CAD build for the part. Positions are in the model's coordinates, mm. A direction names the side the tool comes from. Coordinates: 2 decimals unless noted, no trailing zeros. Loops run counter-clockwise (first coordinate to the right, second up) from the corner with the lowest first, then second, coordinate; pieces in that order, holes last. Notation, with made-up numbers: (-8.75, 21.25) -> (19.25, 21.25) arc R32 ccw to (19.25, 50.25) -> close; hole circle Ø6 at (-32.75, 0). An arc over 180 degrees is marked (long way). Write item = value, one per line. Start each with the question number.
(1) Pull direction Z, two halves, no side cores. Call faces 1 (the face through (3, 6, -8.746)), 2 (the face through (4, 6, -12)), 3 (the face through (4, 0, -13.246)): +Z half, -Z half, draft (parallel to the pull), parting line (faces both ways), or undercut.
(2) Drill centre lines: line 1 (X direction, y = -2, z = -0.75); line 2 (X direction, y = -1.5, z = -3.25); line 3 (Z direction, x = 6, y = 5.5). Where is each one in solid material? Low to high. Write a range as from..to.
(3) Band-saw the part on B-B (x = 3). Write the cut outline in (y, z).
(4) Band-saw the part on D-D (y = -2). Write the cut outline in (x, z).
(5) Band-saw the part on A-A (y = 5.75). Write the cut outline in (x, z).
(6) Flat gauge pins, fed straight in: P1, Ø5, axis at y = -4.5, z = -3, coming from the -X side; P2, Ø1, axis at y = -1, z = -8.5, coming from the -X side; P3, Ø4, axis at x = 11.5, y = 0, coming from the -Z side; P4, Ø1, axis at x = 3, z = -9.5, coming from the +Y side. Where does each tip first touch, or does it go through?
(7) Tool access for faces 4 (the face through (17.5, 0, -1)), 5 (the face through (2, 0, -7)), 6 (the face through (6, 0, -11)), 7 (the face through (8, 0, 0)), 8 (the face through (3, -6, -11.246)): list every direction of +Z, -Z, +X, -X, +Y, -Y with a clear straight run to the whole face (end or side of a thin tool).
(8) Band-saw the part on C-C (z = -9.25). Write the cut outline in (x, y) (1 decimal), and give its area (3 significant figures).
```python
from build123d import *

# Parameters (mm, degrees)
BOSS_EXTRUDE1_DEPTH = 7.5
SKETCH2_W           = 2.5
SKETCH2_H           = 3
CUT_EXTRUDE2_DEPTH  = 20
BOSS_EXTRUDE2_REACH = 16


with BuildPart() as part:
    # Sketch1 → Boss-Extrude1 (new body, symmetric)
    with BuildSketch(Plane(origin=(0, 0, 0), x_dir=(1, 0, 0), z_dir=(0, 1, 0))):
        Polygon((2, 13.245621125), (2, 1.5), (0, 1.5), (0, 0), (15.5, 0), (15.5, -0.754378875), (17.5, -0.754378875), (17.5, 1.128157441), (17.5, 2.995621125), (19, 2.995621125), (19, 4.67916542), (4, 8.745621125), (4, 13.245621125), align=None)
    extrude(amount=BOSS_EXTRUDE1_DEPTH, both=True)

    # Sketch2 → Cut-Extrude2 (cut, through all)
    with BuildSketch(Plane(origin=(0, 0, 0), x_dir=(0, 0, -1), z_dir=(1, 0, 0))):
        with Locations((9.995621125, 6)):
            Rectangle(SKETCH2_W, SKETCH2_H)
        with Locations((9.995621125, -6)):
            Rectangle(SKETCH2_W, SKETCH2_H)
    extrude(amount=CUT_EXTRUDE2_DEPTH, mode=Mode.SUBTRACT)

    # Boss-Extrude2: up to this face of the body (flat: up to its plane)
    boss_extrude2_end = Plane(part.part.faces().sort_by_distance((11.5, 0, -6.712393272))[0])
    # Sketch4 → Boss-Extrude2 (add, up to the picked face)
    with BuildSketch(Plane(origin=(0, 0, -13.245621125), x_dir=(-1, 0, 0), z_dir=(0, 0, -1)), mode=Mode.PRIVATE) as boss_extrude2_sk1:
        with BuildLine():
            Line((-4, 4.5), (-4, -4.5))
            ThreePointArc((-4, -4.5), (-6, 0), (-4, 4.5))
        make_face()
    boss_extrude2_tool1 = split(extrude(boss_extrude2_sk1.sketch, amount=-BOSS_EXTRUDE2_REACH, mode=Mode.PRIVATE), bisect_by=boss_extrude2_end, keep=Keep.BOTH, mode=Mode.PRIVATE)
    add(boss_extrude2_tool1.solids().sort_by_distance((4.812513, 0, -13.245621))[0])


solid = part.part
```
Findings below:
q1.face_1 = undercut
q1.face_2 = draft
q1.face_3 = -Z half
q2.line_1 = 0..17.5
q2.line_2 = 2..19
q2.line_3 = -8.2..0
q3.outline = (-7.5, -13.25) -> (7.5, -13.25) -> (7.5, -11.25) -> (4.5, -11.25) -> (4.5, -8.75) -> (7.5, -8.75) -> (7.5, 0) -> (-7.5, 0) -> (-7.5, -8.75) -> (-4.5, -8.75) -> (-4.5, -11.25) -> (-7.5, -11.25) -> close
q4.outline = (0, -1.5) -> (2, -1.5) -> (2, -13.25) -> (5.66, -13.25) -> (5.66, -8.3) -> (19, -4.68) -> (19, -3) -> (17.5, -3) -> (17.5, 0.75) -> (15.5, 0.75) -> (15.5, 0) -> (0, 0) -> close
q5.outline = (0, -1.5) -> (2, -1.5) -> (2, -8.75) -> (4, -8.75) -> (19, -4.68) -> (19, -3) -> (17.5, -3) -> (17.5, 0.75) -> (15.5, 0.75) -> (15.5, 0) -> (0, 0) -> close; (2, -13.25) -> (4, -13.25) -> (4, -11.25) -> (2, -11.25) -> close
q6.P1 = 0
q6.P2 = 2
q6.P3 = -7.25
q6.P4 = 4.5
q7.face_4 = +Z, +X, +Y, -Y
q7.face_5 = -Z, -X, +Y, -Y
q7.face_6 = -Z, +X
q7.face_7 = +Z, -X, +Y, -Y
q7.face_8 = +X, -X, -Y
q8.outline = (2, -4.5) -> (4, -4.5) arc R6.1 ccw to (4, 4.5) -> (2, 4.5) -> close
q8.area = 30.5 mm²
